from build123d import *

# Parameters (mm, degrees)
SKETCH1_W                                  = 110
SKETCH1_H                                  = 55
SKETCH1_W_2                                = 100
SKETCH1_H_2                                = 45
BOSS_EXTRUDE1_DEPTH                        = 3
BOSS_EXTRUDE2_START                        = -3
SKETCH2_R                                  = 2.75
BOSS_EXTRUDE2_DEPTH                        = 10
MIRROR1_START                              = -3
MIRROR1_AT_THE_SECOND_PLANE_COPY_1_SKETC_R = 2.75
MIRROR1_AT_THE_SECOND_PLANE_COPY_1_DEPTH   = 10


with BuildPart() as part:
    # Sketch1 → Boss-Extrude1 (new body)
    with BuildSketch(Plane(origin=(0, 0, 0), x_dir=(1, 0, 0), z_dir=(0, 1, 0))):
        Rectangle(SKETCH1_W, SKETCH1_H)
        Rectangle(SKETCH1_W_2, SKETCH1_H_2, mode=Mode.SUBTRACT)
    extrude(amount=BOSS_EXTRUDE1_DEPTH)

    # Sketch2 → Boss-Extrude2 (add)
    with BuildSketch(Plane(origin=(0, 3, 0), x_dir=(1, 0, 0), z_dir=(0, 1, 0)).offset(BOSS_EXTRUDE2_START)):
        with BuildLine():
            Line((-50, -22.5), (-42, -22.5))
            Line((-42, -22.5), (-42, -19.889949494))
            ThreePointArc((-42, -19.889949494), (-43.578679656, -16.078679656), (-47.389949494, -14.5))
            Line((-47.389949494, -14.5), (-50, -14.5))
            Line((-50, -14.5), (-50, -22.5))
        make_face()
        with Locations(Location((-45.7, -18.2, 0), (0, 0, 270))):
            Circle(SKETCH2_R, mode=Mode.SUBTRACT)
    boss_extrude2 = extrude(amount=BOSS_EXTRUDE2_DEPTH)

    # Mirror1: Boss-Extrude2 across plane
    add(boss_extrude2.mirror(Plane.XY))

    # Mirror1 at the second plane: Boss-Extrude2 across plane
    add(boss_extrude2.mirror(Plane(origin=(0, 0, 0), x_dir=(0, 0, 1), z_dir=(1, 0, 0))))

    # Mirror1 at the second plane copy 1 sketc → Mirror1 at the second plane copy 1 (add)
    with BuildSketch(Plane(origin=(0, 3, 0), x_dir=(-1, 0, 0), z_dir=(0, 1, 0)).offset(MIRROR1_START)):
        with BuildLine():
            Line((-50, -22.5), (-42, -22.5))
            Line((-42, -22.5), (-42, -19.889949494))
            ThreePointArc((-42, -19.889949494), (-43.578679656, -16.078679656), (-47.389949494, -14.5))
            Line((-47.389949494, -14.5), (-50, -14.5))
            Line((-50, -14.5), (-50, -22.5))
        make_face()
        with Locations(Location((-45.7, -18.2, 0), (0, 0, 270))):
            Circle(MIRROR1_AT_THE_SECOND_PLANE_COPY_1_SKETC_R, mode=Mode.SUBTRACT)
    extrude(amount=MIRROR1_AT_THE_SECOND_PLANE_COPY_1_DEPTH)


solid = part.part
Can you work these out from the model? Positions are in its coordinate system, mm. A direction names the side the tool comes from. Coordinates: 2 decimals unless noted, no trailing zeros. Order: outer loops, then holes, each group sorted by start corner. A loop starts at its lowest first (then second) coordinate and runs counter-clockwise, first axis right, second up. Notation, with made-up numbers: (5, 32.5) -> (61, 32.5) arc R21 cw to (61, 38.5) -> close; hole circle Ø7 at (64, 53.5). An arc over 180 degrees is marked (long way). Use one line per item in the form item = value.
Q1. Imagine slicing it at A-A, the plane y = 5.75. List the corners of the cut face in (x, z) for me.
From the geometry:
outline = (-50, -22.5) -> (-42, -22.5) -> (-42, -19.89) arc R5.39 ccw to (-47.39, -14.5) -> (-50, -14.5) -> close; (-50, 14.5) -> (-47.39, 14.5) arc R5.39 ccw to (-42, 19.89) -> (-42, 22.5) -> (-50, 22.5) -> close; (42, -22.5) -> (50, -22.5) -> (50, -14.5) -> (47.39, -14.5) arc R5.39 ccw to (42, -19.89) -> close; (42, 19.89) arc R5.39 ccw to (47.39, 14.5) -> (50, 14.5) -> (50, 22.5) -> (42, 22.5) -> close; hole circle Ø5.5 at (-45.7, -18.2); hole circle Ø5.5 at (-45.7, 18.2); hole circle Ø5.5 at (45.7, -18.2); hole circle Ø5.5 at (45.7, 18.2)
Q2. Imagine slicing it at B-B, the plane y = 1. List the corners of the cut face in (x, z) for me, then the cut area to 3 significant figures.
From the geometry:
outline = (-55, -27.5) -> (55, -27.5) -> (55, 27.5) -> (-55, 27.5) -> close; hole (-50, -14.5) -> (-47.39, -14.5) arc R5.39 cw to (-42, -19.89) -> (-42, -22.5) -> (42, -22.5) -> (42, -19.89) arc R5.39 cw to (47.39, -14.5) -> (50, -14.5) -> (50, 14.5) -> (47.39, 14.5) arc R5.39 cw to (42, 19.89) -> (42, 22.5) -> (-42, 22.5) -> (-42, 19.89) arc R5.39 cw to (-47.39, 14.5) -> (-50, 14.5) -> close; hole circle Ø5.5 at (-45.7, -18.2); hole circle Ø5.5 at (-45.7, 18.2); hole circle Ø5.5 at (45.7, -18.2); hole circle Ø5.5 at (45.7, 18.2)
area = 1,690 mm²
Q3. We'd pull the mould along X, two halves only. Please class faces 1 (the face through (-50, 6, -18)), 2 (the face through (-48.385, 4.93, -17.604)), 3 (the face through (-4, 0, 23)): released by +X, released by -X, zero draft, split by the parting line, or undercut.
From the geometry:
face_1 = released by -X
face_2 = undercut
face_3 = zero draft
Q4. Imagine slicing it at D-D, the plane x = -45.7. List the corners of the cut face in (y, z) for me.
From the geometry:
outline = (0, -27.5) -> (3, -27.5) -> (3, -22.5) -> (10, -22.5) -> (10, -20.95) -> (0, -20.95) -> close; (0, -15.45) -> (10, -15.45) -> (10, -14.77) -> (0, -14.77) -> close; (0, 14.77) -> (10, 14.77) -> (10, 15.45) -> (0, 15.45) -> close; (0, 20.95) -> (10, 20.95) -> (10, 22.5) -> (3, 22.5) -> (3, 27.5) -> (0, 27.5) -> close
Q5. Will these pins go through, and if not, where does the flat tip stop? P1, Ø5.5, axis at x = 46.5, y = 7.5, coming from the +Z side; P2, Ø3.5, axis at x = -46.5, y = 6, coming from the -Z side; P3, Ø1.3, axis at y = 4, z = -21, coming from the -X side.
From the geometry:
P1 = 22.5
P2 = -22.5
P3 = -50
Q6. I need wall thicknesses on L1, parallel to Z at x = 45.7, y = 2.25; L2, parallel to X at y = 5.5, z = 18; L3, parallel to X at y = 2.75, z = -8. Which ranges of each line are inside material? Lowest first, please.
From the geometry:
L1 = -27.5 to -20.95, -15.45 to -14.77, 14.77 to 15.45, 20.95 to 27.5
L2 = -50 to -48.44, -42.96 to -42.34, 42.34 to 42.96, 48.44 to 50
L3 = -55 to -50, 50 to 55
Q7. Imagine slicing it at C-C, the plane z = -13.5. List the corners of the cut face in (x, y) for me.
From the geometry:
outline = (-55, 0) -> (-50, 0) -> (-50, 3) -> (-55, 3) -> close; (50, 0) -> (55, 0) -> (55, 3) -> (50, 3) -> close
Q8. Which directions (+Z, -Z, +X, -X, +Y, -Y) give clear straight access to the entire face, cutting with the end or side of a thin tool? Please do faces 4 (the face through (-1, 1, 27.5)), 5 (the face through (-42, 5, -21)), 6 (the face through (50, 6, -18)), 7 (the face through (-50, 6, 18)), 8 (the face through (-46, 6, -22.5)).
From the geometry:
face_4 = +Z, +X, -X, +Y, -Y
face_5 = +Y, -Y
face_6 = +Z, -Z, +X, +Y
face_7 = +Z, -Z, -X, +Y
face_8 = -Z, +X, -X, +Y
